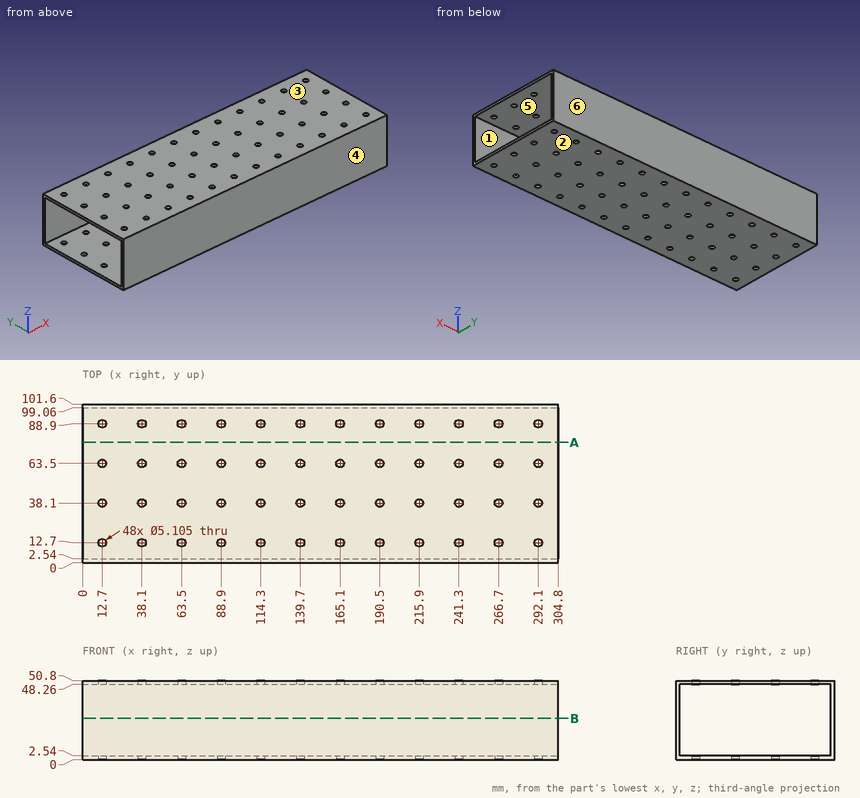
Design review of the part shown in the three views and the two pictorial views. Dimensions are in mm from the part's minimum x, y and z. A direction names the side the tool comes from. Round coordinates to 2 decimals unless told otherwise and drop trailing zeros. Write each loop counter-clockwise with the first axis right and the second up, starting at its lowest first coordinate (ties: lowest second). Pieces come first, ordered by that corner, then holes. Notation, with made-up numbers: M -11.5,53.25 L 6.5,53.25 A17 ccw 6.5,74.25 Z; hole C 82.25,20 d8. An arc over 180 degrees is marked long. Use a Markdown table: item, result. Add a question column.
Q1. We need section A-A, the plane y = 77. State the section outline as (x, z) points.
Q2. The part is to be moulded in two halves that separate along Y. For the marked faces 3, 4, 5 and 6, say which applies: pulls with the +Y half, pulls with the -Y half, needs draft (parallel to the pull), parting line crosses it, or undercut.
Q3. We need section B-B, the plane z = 26.5. State the section outline as (x, y) points.
Q4. Insertion check: pin 1 (4 mm diameter, centred on x = 241.3, y = 88.9, fed in from +Z). The pin has a flat end and moves straight along its axis. Give the tip position at first contact, or say it passes through.
Q5. Machinability: for the marked faces 1 and 2, which of the approach directions +Z, -Z, +X, -X, +Y, -Y give a long, thin tool a straight path to every point of the face, cutting with its end or side? Answer none if there is none.
Q6. To check wall thickness, follow line 1 (Y direction, x = 139.7, z = 0.6); line 2 (Y direction, x = 85, z = 36.5); line 3 (Z direction, x = 72.5, y = 22). State the ranges of each line that lie inside material, in increasing order.
Findings below:
| question | item | result |
|---|---|---|
| 1 | outline | M 0,0 L 304.8,0 L 304.8,2.54 L 0,2.54 Z; M 0,48.26 L 304.8,48.26 L 304.8,50.8 L 0,50.8 Z |
| 2 | face 3 | needs draft |
| 2 | face 4 | pulls with the -Y half |
| 2 | face 5 | undercut |
| 2 | face 6 | pulls with the +Y half |
| 3 | outline | M 0,0 L 304.8,0 L 304.8,2.54 L 0,2.54 Z; M 0,99.06 L 304.8,99.06 L 304.8,101.6 L 0,101.6 Z |
| 4 | pin 1 | passes through |
| 5 | face 1 | +X, -X |
| 5 | face 2 | -Z, +X, -X, +Y, -Y |
| 6 | line 1 | y = 0 to 10.15, 15.25 to 35.55, 40.65 to 60.95, 66.05 to 86.35, 91.45 to 101.6 |
| 6 | line 2 | y = 0 to 2.54, 99.06 to 101.6 |
| 6 | line 3 | z = 0 to 2.54, 48.26 to 50.8 |
